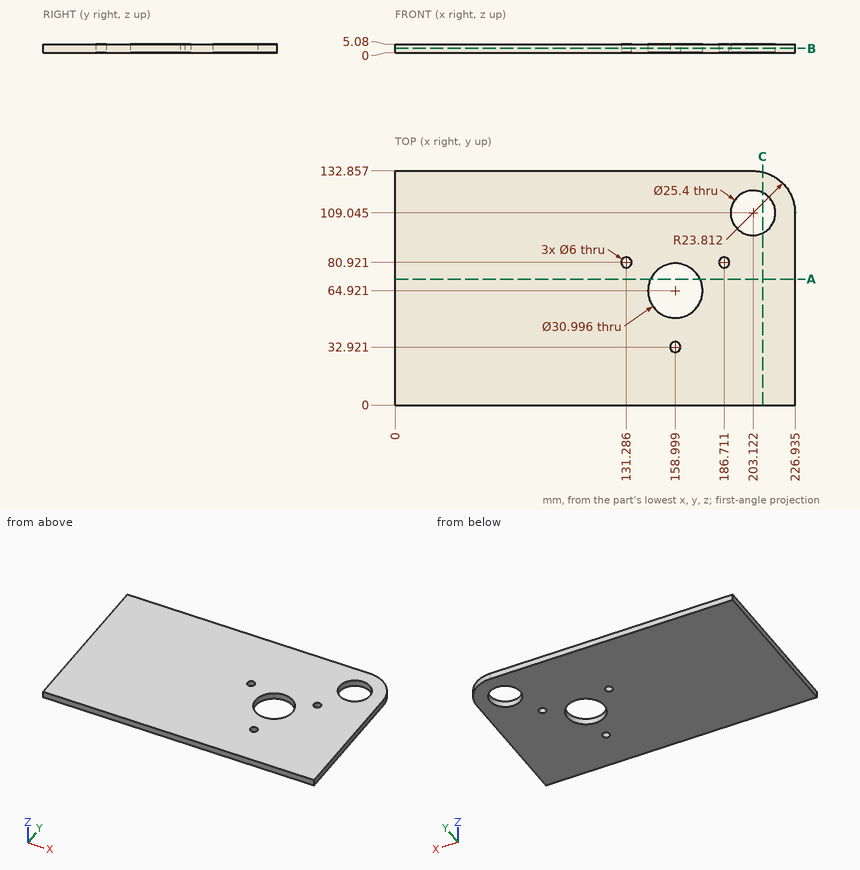
Geometry check sheet. Reference: drawing and pictorial views, mm from the part's lowest x, y, z. Round coordinates to 2 decimals unless told otherwise and drop trailing zeros. Loops run counter-clockwise (first coordinate to the right, second up) from the corner with the lowest first, then second, coordinate; pieces in that order, holes last. Notation, with made-up numbers: (59, 71) -> (98, 71) arc R21 cw to (98, 93) -> close; hole circle Ø6 at (77, 40.25). An arc over 180 degrees is marked (long way). Answer as a JSON object with one key per item and string values. Group by question number.
Item 1: Cross-section at C-C, the plane x = 208.5. Record the cut outline in (y, z), plus the area to 3 significant figures.
Item 2: Cross-section at A-A, the plane y = 71.5. Record the cut outline in (x, z) (1 decimal).
Item 3: Thickness scan on line 1 along Y through (x, z) = (157.5, 3.3) (1 decimal); line 2 along Y through (x, z) = (171, 3.25) (1 decimal); line 3 along Y through (x, z) = (186.5, 0.5) (1 decimal). Record the ranges inside material, lowest first.
Item 4: Cross-section at B-B, the plane z = 2.6. Record the cut outline in (x, y) (1 decimal), plus the area to 3 significant figures.
Determined:
{
 "1": {"outline": "(0, 0) -> (97.54, 0) -> (97.54, 5.08) -> (0, 5.08) -> close; (120.55, 0) -> (132.24, 0) -> (132.24, 5.08) -> (120.55, 5.08) -> close", "area": "555 mm²"},
 "2": {"outline": "(0, 0) -> (145, 0) -> (145, 5.1) -> (0, 5.1) -> close; (173, 0) -> (226.9, 0) -> (226.9, 5.1) -> (173, 5.1) -> close"},
 "3": {"line 1": "y = 0 to 30.3, 35.5 to 49.5, 80.3 to 132.9", "line 2": "y = 0 to 55.1, 74.7 to 132.9", "line 3": "y = 0 to 77.9, 83.9 to 132.9"},
 "4": {"outline": "(0, 0) -> (226.9, 0) -> (226.9, 109) arc R23.8 ccw to (203.1, 132.9) -> (0, 132.9) -> close; hole circle Ø6 at (131.3, 80.9); hole circle Ø31 at (159, 64.9); hole circle Ø6 at (159, 32.9); hole circle Ø6 at (186.7, 80.9); hole circle Ø25.4 at (203.1, 109)", "area": "28,700 mm²"}
}
